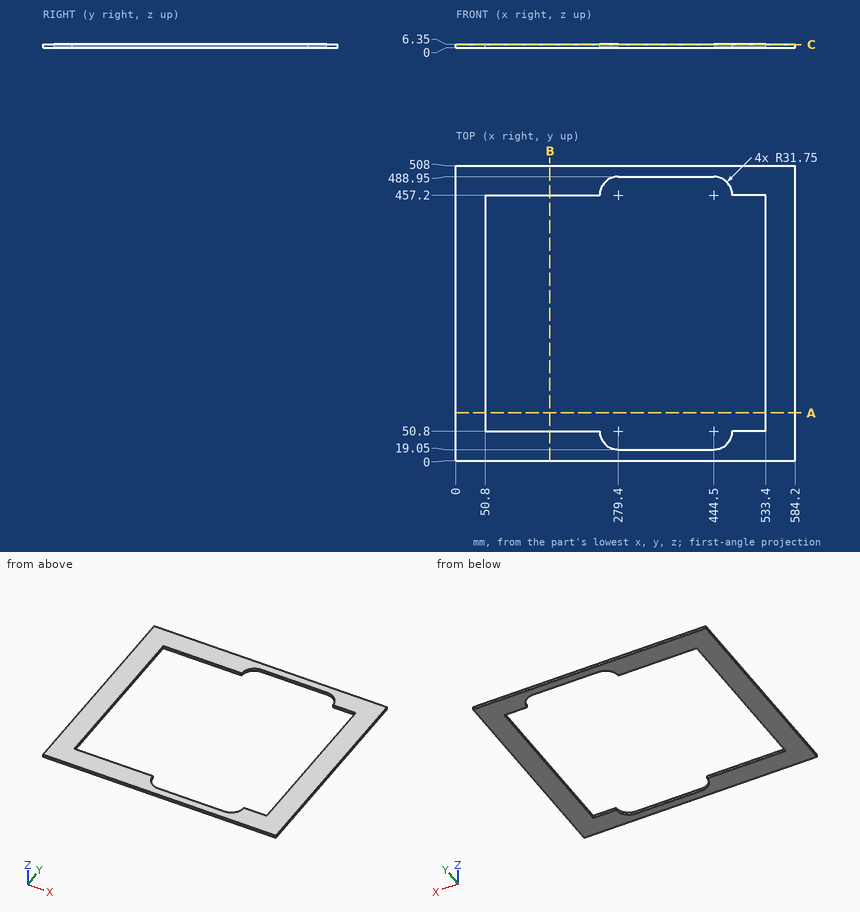
Part print with two shaded views. Sizes in mm from the minimum x, y, z corner. Coordinates: 2 decimals unless noted, no trailing zeros. Write each loop counter-clockwise with the first axis right and the second up, starting at its lowest first coordinate (ties: lowest second). Pieces come first, ordered by that corner, then holes. Notation, with made-up numbers: (-28, 2) - (30, 2) arc R15 ccw to (30, 30) - close; hole circle Ø10 at (-1.75, 2). An arc over 180 degrees is marked (long way). Put each result on its own line as item: value.
1. Band-saw the part on B-B (x = 162). Write the cut outline in (y, z), then the cut area to 3 significant figures.
Final values:
outline: (0, 0) - (50.8, 0) - (50.8, 6.35) - (0, 6.35) - close; (457.2, 0) - (508, 0) - (508, 6.35) - (457.2, 6.35) - close
area: 645 mm²
2. Band-saw the part on C-C (z = 5.25). Write the cut outline in (x, y), then the cut area to 3 significant figures.
Final values:
outline: (0, 0) - (584.2, 0) - (584.2, 508) - (0, 508) - close; hole (50.8, 50.8) - (247.65, 50.8) arc R31.75 ccw to (279.4, 19.05) - (444.5, 19.05) arc R31.75 ccw to (476.25, 50.8) - (533.4, 50.8) - (533.4, 457.2) - (476.25, 457.2) arc R31.75 ccw to (444.5, 488.95) - (279.4, 488.95) arc R31.75 ccw to (247.65, 457.2) - (50.8, 457.2) - close
area: 87,000 mm²
3. Band-saw the part on A-A (y = 82). Write the cut outline in (x, z).
Final values:
outline: (0, 0) - (50.8, 0) - (50.8, 6.35) - (0, 6.35) - close; (533.4, 0) - (584.2, 0) - (584.2, 6.35) - (533.4, 6.35) - close
4. Probe line 1 along Y through (x, z) = (52.5, 4.75); line 2 along Y through (x, z) = (434.5, 0.5); line 3 along X through (y, z) = (285, 0.5). List the from-to ranges inside material, lowest first. Write a range as [from, to].
Final values:
line 1: y = [0, 50.8], [457.2, 508]
line 2: y = [0, 19.05], [488.95, 508]
line 3: x = [0, 50.8], [533.4, 584.2]
